Geometry check sheet. Reference: the model listing, model coordinates, mm. Coordinates: 2 decimals unless noted, no trailing zeros. Write each loop counter-clockwise with the first axis right and the second up, starting at its lowest first coordinate (ties: lowest second). Pieces come first, ordered by that corner, then holes. Notation, with made-up numbers: (45, -17) -> (102, -17) arc R5 cw to (102, -8) -> close; hole circle Ø10 at (75, 49.5). An arc over 180 degrees is marked (long way). Answer in a Markdown table with one row per item. Add a question column.
1. Depth check by flat-ended pin: P1, Ø2.5, axis at x = -30, z = -170, coming from the +Y side. Enter the tip coordinate at first touch or a pass-through.
2. Cross-section at B-B on y = 2.3. Give the number of separate pieces and of enclosed holes in the cut face, and give its area (3 significant figures).
3. Cross-section at A-A on z = -142. Record the cut outline in (x, y).
4. Scan line: L1, parallel to X at y = 0.45, z = 86. Record every from-to range of solid material in increasing order. Write a range as from..to.
```python
from build123d import *

# Parameters (mm, degrees)
SKETCH1_W           = 120
SKETCH1_H           = 360
BOSS_EXTRUDE1_DEPTH = 3
SKETCH2_R           = 2
CUT_EXTRUDE2_DEPTH  = 190.76037521
CUT_EXTRUDE3_DEPTH  = 190.76037521


with BuildPart() as part:
    # Sketch1 → Boss-Extrude1 (new body)
    with BuildSketch(Plane(origin=(0, 0, 0), x_dir=(1, 0, 0), z_dir=(0, 1, 0))):
        Rectangle(SKETCH1_W, SKETCH1_H)
    extrude(amount=BOSS_EXTRUDE1_DEPTH)

    # Sketch2 → Cut-Extrude2 (cut, through all)
    with BuildSketch(Plane(origin=(0, 3, 0), x_dir=(1, 0, 0), z_dir=(0, 1, 0))):
        with Locations(Location((-30, 170, 0), (0, 0, 270))):
            Circle(SKETCH2_R)
        with Locations(Location((30, 170, 0), (0, 0, 270))):
            Circle(SKETCH2_R)
        with Locations(Location((-30, -170, 0), (0, 0, 270))):
            Circle(SKETCH2_R)
        with Locations(Location((30, -170, 0), (0, 0, 270))):
            Circle(SKETCH2_R)
        with Locations(Location((-30, 25, 0), (0, 0, 270))):
            Circle(SKETCH2_R)
        with Locations(Location((30, 25, 0), (0, 0, 270))):
            Circle(SKETCH2_R)
        with Locations(Location((-30, -25, 0), (0, 0, 270))):
            Circle(SKETCH2_R)
        with Locations(Location((30, -25, 0), (0, 0, 270))):
            Circle(SKETCH2_R)
    extrude(amount=-CUT_EXTRUDE2_DEPTH, mode=Mode.SUBTRACT)

    # Sketch3 → Cut-Extrude3 (cut, through all)
    with BuildSketch(Plane(origin=(0, 3, 0), x_dir=(1, 0, 0), z_dir=(0, 1, 0))):
        with BuildLine():
            Line((32, 150), (32, 50))
            ThreePointArc((32, 50), (30, 48), (28, 50))
            Line((28, 50), (28, 150))
            ThreePointArc((28, 150), (30, 152), (32, 150))
        make_face()
        with BuildLine():
            Line((-28, 150), (-28, 50))
            ThreePointArc((-28, 50), (-30, 48), (-32, 50))
            Line((-32, 50), (-32, 150))
            ThreePointArc((-32, 150), (-30, 152), (-28, 150))
        make_face()
        with BuildLine():
            Line((28, -150), (28, -50))
            ThreePointArc((28, -50), (30, -48), (32, -50))
            Line((32, -50), (32, -150))
            ThreePointArc((32, -150), (30, -152), (28, -150))
        make_face()
        with BuildLine():
            Line((-32, -150), (-32, -50))
            ThreePointArc((-32, -50), (-30, -48), (-28, -50))
            Line((-28, -50), (-28, -150))
            ThreePointArc((-28, -150), (-30, -152), (-32, -150))
        make_face()
    extrude(amount=-CUT_EXTRUDE3_DEPTH, mode=Mode.SUBTRACT)


solid = part.part
```
Results found:
| question | item | result |
|---|---|---|
| 1 | P1 | passes through |
| 2 | separate pieces | 1 |
| 2 | enclosed holes | 12 |
| 2 | area | 41,400 mm^2 |
| 3 | outline | (-60, 0) -> (-32, 0) -> (-32, 3) -> (-60, 3) -> close; (-28, 0) -> (28, 0) -> (28, 3) -> (-28, 3) -> close; (32, 0) -> (60, 0) -> (60, 3) -> (32, 3) -> close |
| 4 | L1 | x = -60..-32, -28..28, 32..60 |
